The model under review builds one solid part; all positions refer to its coordinate system, in mm. Coordinates: 2 decimals unless noted, no trailing zeros. Order: outer loops, then holes, each group sorted by start corner. A loop starts at its lowest first (then second) coordinate and runs counter-clockwise, first axis right, second up.
from build123d import *

# Parameters (mm, degrees)
F0_W     = 99.9998
F0_H     = 46.00928
F1_DEPTH = 25.4
F2_R     = 8.255
F3_DEPTH = 127


with BuildPart() as f1:
    # F0 (on Top) → F1 (new body)
    with BuildSketch(Plane.XY):
        Rectangle(F0_W, F0_H)
    extrude(amount=F1_DEPTH)

    # F2 (on Front) → F3 (cut, symmetric)
    with BuildSketch(Plane.XZ):
        with Locations((-29.9974, 25.907155)):
            Circle(F2_R)
        with Locations((29.9974, 25.907155)):
            Circle(F2_R)
    extrude(amount=F3_DEPTH, both=True, mode=Mode.SUBTRACT)


solid = f1.part
(1) The part is to be moulded in two halves that separate along X. For faces 1 (the face through (0, 0, 25.4)), 2 (the face through (29.823, -0.322, 17.654)), 3 (the face through (50, 0, 13)), 4 (the face through (-30.172, 0.322, 17.654)), say which applies: +X half, -X half, draft (parallel to the pull), parting line (faces both ways), or undercut.
(2) Consider section C-C (z = 23.5). Give the boundary of the cut face in (x, y), then the cut area to 3 significant figures.
(3) Consider section B-B (y = 19). Give the boundary of the cut face in (x, z) (3 decimals), then the cut area to 3 significant figures.
(4) Consider section D-D (x = 23). Give the boundary of the cut face in (y, z), then the cut area to 3 significant figures.
(5) Wall thickness on line 1 (X direction, y = -18, z = 20); line 2 (X direction, y = -9, z = 20.5) (3 decimals); line 3 (Z direction, x = 34.5, y = -3.5): over which ranges is each line inside the solid? List them lowest first.
(6) Consider section A-A (z = 19). Give the boundary of the cut face in (x, y).
(7) Insertion check: pin 1 Ø4 at (x, y) = (28.5, -9.5) entering from -Z. The pin has a flat end and moves straight along its axis. Give the tip position at first contact, or say it passes through.
Findings:
1. face 1: draft
1. face 2: undercut
1. face 3: +X half
1. face 4: undercut
2. outline: (-50, -23) - (-37.89, -23) - (-37.89, 23) - (-50, 23) - close; (-22.1, -23) - (22.1, -23) - (22.1, 23) - (-22.1, 23) - close; (37.89, -23) - (50, -23) - (50, 23) - (37.89, 23) - close
2. area: 3,150 mm2
3. outline: (-50, 0) - (50, 0) - (50, 25.4) - (38.237, 25.4) arc R8.255 cw to (21.758, 25.4) - (-21.758, 25.4) arc R8.255 cw to (-38.237, 25.4) - (-50, 25.4) - close
3. area: 2,340 mm2
4. outline: (-23, 0) - (23, 0) - (23, 21.53) - (-23, 21.53) - close
4. area: 990 mm2
5. line 1: x = -50 to -35.76, -24.23 to 24.23, 35.76 to 50
5. line 2: x = -50 to -36.235, -23.76 to 23.76, 36.235 to 50
5. line 3: z = 0 to 18.99
6. outline: (-50, -23) - (-34.52, -23) - (-34.52, 23) - (-50, 23) - close; (-25.48, -23) - (25.48, -23) - (25.48, 23) - (-25.48, 23) - close; (34.52, -23) - (50, -23) - (50, 23) - (34.52, 23) - close
7. pin 1: stops at z = 0
